Autodesk Inventor part; units mm, degrees
ref_plane "YZ Plane" through (0, 0, 0) normal (1, 0, 0) x (0, 1, 0)
ref_plane "XZ Plane" through (0, 0, 0) normal (0, 1, 0) x (-1, 0, 0)
ref_plane "XY Plane" through (0, 0, 0) normal (0, 0, 1) x (1, 0, 0)
sketch "Sketch1" plane through (0, 0, 0) normal (1, 0, 0) x (0, 1, 0)
  line L0 (9.25, -16.5) -> (11.25, -16.5)
  line L1 (11.25, -16.5) -> (11.25, 2)
  line L2 (11.25, 2) -> (-11.25, 2)
  line L3 (-11.25, 2) -> (-11.25, -16.5)
  line L4 (-11.25, -16.5) -> (-9.25, -16.5)
  line L5 (-9.25, -16.5) -> (-9.25, 0)
  line L6 (-9.25, 0) -> (9.25, 0)
  line L7 (9.25, 0) -> (9.25, -16.5)
  point P0 (0, 0)
  point P1 (0, 0)
  point P2 (10.25, -16.5)
  point P3 (-10.25, -16.5)
  dimension "d0" = 18.5
  dimension "d1" = 2
  dimension "d2" = 2
  dimension "d3" = 18.5
extrude "Extrusion1" add sketch "Sketch1" along normal blind 20
sketch "Sketch2" plane through (20, 0, 0) normal (1, 0, 0) x (0, 0, -1)
  line L0 (16.5, 9.25) -> (16.5, 11.25)
  line L1 (16.5, 11.25) -> (-2, 11.25)
  line L2 (-2, 11.25) -> (-2, -11.25)
  line L3 (-2, -11.25) -> (16.5, -11.25)
  line L4 (16.5, -11.25) -> (16.5, -9.25)
  line L5 (16.5, -9.25) -> (0, -9.25)
  line L6 (0, -9.25) -> (0, 9.25)
  line L7 (0, 9.25) -> (16.5, 9.25)
  line L8 (16.5, 9.25) -> (16.5, 11.25)
  line L9 (16.5, 11.25) -> (-2, 11.25)
  line L10 (-2, 11.25) -> (-2, 29.75)
  line L11 (-2, 29.75) -> (16.5, 29.75)
  line L12 (16.5, 29.75) -> (16.5, 11.25)
  point P0 (0, 0)
  dimension "d6" = 18.5
extrude "Extrusion2" add sketch "Sketch2" against normal blind 2 contours L1 L10 L11 L12
sketch "Sketch3" plane through (20, 0, 0) normal (1, 0, 0) x (0, 0, -1)
  line L0 (16.5, 9.25) -> (16.5, 29.75)
  line L1 (16.5, 29.75) -> (-2, 29.75)
  line L2 (-2, 29.75) -> (-2, -11.25)
  line L3 (-2, -11.25) -> (16.5, -11.25)
  line L4 (16.5, -11.25) -> (16.5, -9.25)
  line L5 (16.5, -9.25) -> (0, -9.25)
  line L6 (0, -9.25) -> (0, 9.25)
  line L7 (0, 9.25) -> (16.5, 9.25)
  line L8 (16.5, 29.75) -> (16.5, 15.25)
  line L9 (16.5, 9.25) -> (16.5, 29.75)
  line L10 (16.5, 15.25) -> (18.5, 15.25)
  line L11 (18.5, 15.25) -> (18.5, 29.75)
  line L12 (18.5, 29.75) -> (16.5, 29.75)
  point P0 (0, 0)
  dimension "d9" = 6
  dimension "d10" = 2
extrude "Extrusion3" add sketch "Sketch3" along normal blind 18.5 and the other way blind 2 contours L0 L12 L11 L10
sketch "Sketch4" plane through (0, 0, 0) normal (-1, 0, 0) x (0, 0, 1)
  line L0 (-16.5, 9.25) -> (-16.5, 11.25)
  line L1 (0, 9.25) -> (-16.5, 9.25)
  line L2 (0, -9.25) -> (0, 9.25)
  line L3 (-16.5, -9.25) -> (0, -9.25)
  line L4 (-16.5, -11.25) -> (-16.5, -9.25)
  line L5 (2, -11.25) -> (-16.5, -11.25)
  line L6 (2, 11.25) -> (2, -11.25)
  line L7 (-16.5, 11.25) -> (2, 11.25)
  line L8 (-16.5, -9.25) -> (0, -9.25)
  line L9 (-16.5, -9.25) -> (65.5, -9.25)
  line L10 (65.5, -9.25) -> (65.5, -41.25)
  line L11 (65.5, -41.25) -> (-16.5, -41.25)
  line L12 (-16.5, -41.25) -> (-16.5, -9.25)
  point P0 (0, 0)
  dimension "d15" = 82
  dimension "d16" = 30
extrude "Extrusion4" add sketch "Sketch4" against normal blind 3 contours L9 L6 L5 L4 L3 | L9 L10 L11 L12 L5 L6
sketch "Sketch5" plane through (3, 0, 0) normal (1, 0, 0) x (0, 0, -1)
  line L0 (-2, -9.25) -> (-2, -11.25)
  line L1 (-2, -9.25) -> (-65.5, -9.25)
  line L2 (-65.5, -9.25) -> (-65.5, -41.25)
  line L3 (-65.5, -41.25) -> (16.5, -41.25)
  line L4 (16.5, -41.25) -> (16.5, -11.25)
  line L5 (-2, -11.25) -> (16.5, -11.25)
  arc A0 (16.5, -41.25) -> (-65.5, -41.25) centre (-24.5, -89.7833) ccw
  point P0 (0, 0)
  dimension "d20" = 15
extrude "Extrusion5" add sketch "Sketch5" along normal blind 39 contours A0 L3
sketch "Sketch7" plane through (42, 0, 0) normal (1, 0, 0) x (0, 0, -1)
  line L0 (-65.5, -41.25) -> (16.5, -41.25)
  arc A0 (16.5, -41.25) -> (-65.5, -41.25) centre (-24.5, -89.7833) ccw
  line L1 (-67.5, -41.25) -> (18.5, -41.25)
  arc A1 (18.5, -41.25) -> (-67.5, -41.25) centre (-24.5, -87.1324) ccw
  point P0 (0, 0)
  dimension "d33" = 2
  dimension "d34" = 2
  dimension "d35" = 2
extrude "Extrusion6" add sketch "Sketch7" along normal blind 2
sketch "Sketch8" plane through (44, 0, 0) normal (1, 0, 0) x (0, 0, -1)
  arc A0 (16.5, -41.25) -> (-65.5, -41.25) centre (-24.5, -89.7833) ccw
  line L0 (16.5, -41.25) -> (16.5, -11.25)
  line L1 (-2, -11.25) -> (16.5, -11.25)
  line L2 (-2, -9.25) -> (-2, -11.25)
  line L3 (-2, -9.25) -> (-65.5, -9.25)
  line L4 (-65.5, -9.25) -> (-65.5, -41.25)
  line L5 (-67.5, -41.25) -> (18.5, -41.25)
  arc A1 (18.5, -41.25) -> (-67.5, -41.25) centre (-24.5, -87.1324) ccw
  arc A2 (18.5, -41.25) -> (-67.5, -41.25) centre (-24.5, -87.1324) ccw
  line L6 (-67.5, -41.25) -> (-65.5, -41.25)
  line L7 (-65.5, -41.25) -> (-65.5, -39.4544)
  line L8 (-65.5, -39.4544) -> (-67.5, -39.4544)
  line L9 (-67.5, -39.4544) -> (-67.5, -41.25)
  line L10 (16.5, -41.25) -> (18.5, -41.25)
  line L11 (16.5, -9.25) -> (16.5, -41.25)
  line L12 (18.5, -41.25) -> (16.5, -41.25)
  line L13 (16.5, -41.25) -> (16.5, -39.4544)
  line L14 (16.5, -39.4544) -> (18.5, -39.4544)
  line L15 (18.5, -39.4544) -> (18.5, -41.25)
  point P0 (0, 0)
extrude "Extrusion7" cut sketch "Sketch8" against normal up to surface (2 mm away) contours L0 A1 L5 | L5 A1 L4
fillet "Fillet1" radius 1 9 edges at (3, -26.25, 24.5) (20, 22.5, -16.5) (1.5, -9.25, 2) (3, -10.25, 2) (3, -11.25, -7.25) (10, 9.25, 0) (10, -9.25, 0) (18, 11.25, -7.25) (19, 15.25, -16.5)
equation "\"d2\" = d1"
equation "\"d3\" = d0"
equation "\"d34\" = d33"
properties part number "headphonesDeskHanger"
CAD build for the part. Positions are in the model's coordinates, mm. A direction names the side the tool comes from. Round coordinates to 2 decimals unless told otherwise and drop trailing zeros. Order: outer loops, then holes, each group sorted by start corner. A loop starts at its lowest first (then second) coordinate and runs counter-clockwise, first axis right, second up.
Q1. Drop flat-ended pins along their axis: pin 1 (4 mm diameter, centred on x = 14, y = -5.5, fed in from +Z); pin 2 (5 mm diameter, centred on x = 29.5, y = -22, fed in from +Z); pin 3 (3 mm diameter, centred on y = -12.5, z = -2, fed in from +X); pin 4 (17 mm diameter, centred on x = 8, z = -12.5, fed in from +Y). Give the stop position or say it passes through.
Q2. Slice it at D-D (x = 41). Write the cut outline in (y, z), and give its area (3 significant figures).
Q3. Slice it at C-C (x = 34.5). Write the cut outline in (y, z).
Q4. Wall check: L1, parallel to Y at x = 15.5, z = -14; L2, parallel to X at y = -29, z = 1; L3, parallel to X at y = -11.5, z = 31.5. Give the ranges that are in metal, low to high.
Q5. Two-plate mould, pull along Y, no slides. Class faces 5 (the flat face through (10, 9.25, -9)), 6 (the flat face through (25, 29.75, -17)), 7 (the flat face through (10, 0, 2)): pulls with the +Y half, pulls with the -Y half, needs draft (parallel to the pull), parting line crosses it, or undercut.
Q6. Slice it at A-A (x = 5). Write the cut outline in (y, z).
Q7. Which spindle directions (+Z, -Z, +X, -X, +Y, -Y) get a long thin tool onto all of the face, cutting with end or side? Do faces 1 (the flat face through (1, -9.25, 34)), 2 (the flat face through (30, 22, -16.5)), 3 (the flat face through (8, 11.25, -7)), 4 (the flat face through (10, 0, 0)). Say none if no direction does.
Q8. Slice it at B-B (y = -4). Write the cut outline in (x, z).
Results below:
1. pin 1: stops at z = 2
1. pin 2: passes through
1. pin 3: stops at x = 20
1. pin 4: stops at y = 11.25
2. outline: (-41.25, -16.5) arc R63.53 ccw to (-41.25, 65.5) - close
2. area: 842 mm2
3. outline: (-41.25, -16.5) arc R63.53 ccw to (-41.25, 65.5) - close; (15.25, -18.5) - (29.75, -18.5) - (29.75, -16.5) - (15.25, -16.5) - close
4. L1: y = -41.25 to -39.24, -11.25 to -9.25, 9.25 to 11.25
4. L2: x = 0 to 3, 42 to 44
4. L3: x = 0 to 3
5. face 5: undercut
5. face 6: pulls with the +Y half
5. face 7: needs draft
6. outline: (-41.25, -16.5) arc R63.53 ccw to (-41.25, 65.5) - close; (-11.25, -16.5) - (-9.25, -16.5) - (-9.25, -1) arc R1 cw to (-8.25, 0) - (8.25, 0) arc R1 cw to (9.25, -1) - (9.25, -16.5) - (11.25, -16.5) - (11.25, 2) - (-11.25, 2) - close
7. face 1: +Z, +X, -X, +Y
7. face 2: +Z, +X, +Y
7. face 3: +Z, -Z, -X, +Y
7. face 4: -Z, +X, -X
8. outline: (0, 0) - (20, 0) - (20, 2) - (0, 2) - close
